from build123d import *

# Parameters (mm, degrees)
SKETCH1_R               = 8.189006913
BOSS_EXTRUDE1_DEPTH     = 15
SKETCH2_R               = 3
CUT_EXTRUDE1_DEPTH      = 30
SKETCH4_W               = 1.839212521
SKETCH4_H               = 4.190652527
BOSS_EXTRUDE2_DEPTH     = 10
SKETCH3_R               = 1.5
CUT_EXTRUDE2_DEPTH      = 10
CUT_EXTRUDE2_DEPTH_BACK = 10


with BuildPart() as part:
    # Sketch1 → Boss-Extrude1 (new body)
    with BuildSketch(Plane(origin=(0, 0, 0), x_dir=(1, 0, 0), z_dir=(0, 1, 0))):
        Circle(SKETCH1_R)
    extrude(amount=BOSS_EXTRUDE1_DEPTH)

    # Sketch2 → Cut-Extrude1 (cut)
    with BuildSketch(Plane(origin=(0, 15, 0), x_dir=(1, 0, 0), z_dir=(0, 1, 0))):
        Circle(SKETCH2_R)
    extrude(amount=-CUT_EXTRUDE1_DEPTH, mode=Mode.SUBTRACT)

    # Sketch4 → Boss-Extrude2 (add)
    with BuildSketch(Plane(origin=(0, 15, 0), x_dir=(1, 0, 0), z_dir=(0, 1, 0))):
        with Locations((-3.214713917, 0.163363311)):
            Rectangle(SKETCH4_W, SKETCH4_H)
    extrude(amount=-BOSS_EXTRUDE2_DEPTH)

    # Sketch3 → Cut-Extrude2 (cut, two sides)
    with BuildSketch(Plane(origin=(0, 0, 0), x_dir=(0, 0, -1), z_dir=(1, 0, 0))) as cut_extrude2_sk:
        with Locations((0, 10)):
            Circle(SKETCH3_R)
    extrude(amount=CUT_EXTRUDE2_DEPTH, mode=Mode.SUBTRACT)
    extrude(cut_extrude2_sk.sketch, amount=-CUT_EXTRUDE2_DEPTH_BACK, mode=Mode.SUBTRACT)


solid = part.part
Verification items for the finished model (mm, model axes). Coordinates: 2 decimals unless noted, no trailing zeros. Write each loop counter-clockwise with the first axis right and the second up, starting at its lowest first coordinate (ties: lowest second). Pieces come first, ordered by that corner, then holes. Notation, with made-up numbers: M 53,17 L 91,17 A32 ccw 91,47 Z; hole C 66.5,-24.75 d9. An arc over 180 degrees is marked long. Use CSV: the item, a comma, the result in double quotes.
Q1. Section check D-D, the plane y = 4.5. Enter the section's corners in (x, z), and give its area (3 significant figures).
Computed values:
outline,"C 0,0 d16.38; hole C 0,0 d6"
area,"182 mm²"
Q2. Section check C-C, the plane y = 10. Enter the section's corners in (x, z), and give its area (3 significant figures).
Computed values:
outline,"M -8.05,-1.5 A8.19 ccw 8.05,-1.5 L 2.6,-1.5 A3 cw -2.3,-1.93 L -2.3,-1.5 Z; M -8.05,1.5 L -2.3,1.5 L -2.3,1.93 A3 cw 2.6,1.5 L 8.05,1.5 A8.19 ccw Z"
area,"151 mm²"
Q3. Go/stop test with flat-tipped pins: P1, Ø1, axis at x = 6, y = 10, coming from the -Z side; P2, Ø1, axis at y = 2.5, z = 2, coming from the +X side; P3, Ø0.6, axis at x = -2.5, z = -0.5, coming from the -Y side; P4, Ø1.2, axis at y = 12, z = -0.5, coming from the +X side. Record where each tip stops, or that it passes through.
Computed values:
P1,"z = -6.07"
P2,"x = 8.05"
P3,"y = 5"
P4,"x = 8.19"
Q4. Section check B-B, the plane x = 0. Enter the section's corners in (y, z).
Computed values:
outline,"M 0,-8.19 L 15,-8.19 L 15,-3 L 0,-3 Z; M 0,3 L 15,3 L 15,8.19 L 0,8.19 Z"
Q5. Section check A-A, the plane z = 0. Enter the section's corners in (x, y), and give its area (3 significant figures).
Computed values:
outline,"M -8.19,0 L -3,0 L -3,5 L -2.3,5 L -2.3,8.5 L -8.19,8.5 Z; M -8.19,11.5 L -2.3,11.5 L -2.3,15 L -8.19,15 Z; M 3,0 L 8.19,0 L 8.19,8.5 L 3,8.5 Z; M 3,11.5 L 8.19,11.5 L 8.19,15 L 3,15 Z"
area,"129 mm²"
Q6. Mould release check, pull along Y, two halves, no side actions. Record for faces 1 (the cylindrical face through (-5.201, 8.536, 0.325)), 2 (the flat face through (4, 15, 0)), 3 (the flat face through (-2.295, 8.96, 1.32)): pulls with the +Y half, pulls with the -Y half, needs draft (parallel to the pull), parting line crosses it, or undercut.
Computed values:
face 1,"undercut"
face 2,"pulls with the +Y half"
face 3,"needs draft"
Q7. Thickness scan on line 1 along X through (y, z) = (12.25, 0); line 2 along Y through (x, z) = (4.5, 0); line 3 along X through (y, z) = (2.5, 0). Record the ranges inside material, lowest first. Write a range as [from, to].
Computed values:
line 1,"[-8.19, -2.3], [3, 8.19]"
line 2,"[0, 8.5], [11.5, 15]"
line 3,"[-8.19, -3], [3, 8.19]"
